Part model, mm, in its own coordinate system. Round coordinates to 2 decimals unless told otherwise and drop trailing zeros. Loops run counter-clockwise (first coordinate to the right, second up) from the corner with the lowest first, then second, coordinate; pieces in that order, holes last.
(1) Cut at B-B on y = 4. List the corners of the cut face in (x, z).
(2) Cut at C-C on x = -27. List the corners of the cut face in (y, z).
(3) Mould opens along Z. For faces 1 (the face through (-63, 0, -75)), 2 (the face through (-64, 3, 0)), 3 (the face through (-23.483, 3.219, -32.203)), 4 (the face through (-63, 3, -152.4)) say: +Z half, -Z half, draft (parallel to the pull), parting line (faces both ways), or undercut.
(4) Cut at A-A on z = -50.8. List the corners of the cut face in (x, y).
(5) Probe probe 1 along X at (y, z) = (5, -50.8); probe 2 along Z at (x, y) = (-6, 5.5); probe 3 along X at (y, z) = (1, -61). List the from-to ranges inside material, lowest first.
Autodesk Inventor part; units mm, degrees
ref_plane "YZ Plane" through (0, 0, 0) normal (1, 0, 0) x (0, 1, 0)
ref_plane "XZ Plane" through (0, 0, 0) normal (0, 1, 0) x (-1, 0, 0)
ref_plane "XY Plane" through (0, 0, 0) normal (0, 0, 1) x (1, 0, 0)
sketch "Sketch1" plane through (0, 0, 0) normal (0, 1, 0) x (-1, 0, 0)
  line L0 (0, 0) -> (0, -152.4)
  line L1 (0, -152.4) -> (127, -152.4)
  line L2 (127, -152.4) -> (127, 0)
  line L3 (127, 0) -> (0, 0)
  dimension "d0" = 152.4
  dimension "d1" = 127
extrude "Extrusion1" add sketch "Sketch1" along normal blind 6.35
sketch "Sketch2" plane through (0, 6.35, 0) normal (0, 1, 0) x (1, 0, 0)
  circle A0 centre (-19.3538, 50.8) radius 19.05
  point P0 (0, 0)
  dimension "d5" = 38.1
extrude "Extrusion2" cut sketch "Sketch2" against normal blind 6.35
properties part number "Side_chasis"
Final values:
1. outline: (-127, -152.4) - (0, -152.4) - (0, 0) - (-127, 0) - close; hole circle Ø38.1 at (-19.35, -50.8)
2. outline: (0, -152.4) - (6.35, -152.4) - (6.35, -68.25) - (0, -68.25) - close; (0, -33.35) - (6.35, -33.35) - (6.35, 0) - (0, 0) - close
3. face 1: draft
3. face 2: +Z half
3. face 3: undercut
3. face 4: -Z half
4. outline: (-127, 0) - (-38.4, 0) - (-38.4, 6.35) - (-127, 6.35) - close; (-0.3, 0) - (0, 0) - (0, 6.35) - (-0.3, 6.35) - close
5. probe 1: x = -127 to -38.4, -0.3 to 0
5. probe 2: z = -152.4 to -64.39, -37.21 to 0
5. probe 3: x = -127 to -35.44, -3.26 to 0
